For this review, use the dimensioned drawing (mm, ordinates from the lowest corner) and the shaded views. A direction names the side the tool comes from. Give positions to 0.01 mm unless a question says otherwise; leave off trailing zeros. Order: outer loops, then holes, each group sorted by start corner. A loop starts at its lowest first (then second) coordinate and runs counter-clockwise, first axis right, second up. Notation, with made-up numbers: (13, 72) - (30, 72) arc R29 cw to (30, 110) - close; hole circle Ø9 at (12.25, 70). An arc over 180 degrees is marked (long way). One line per item, written item: value.
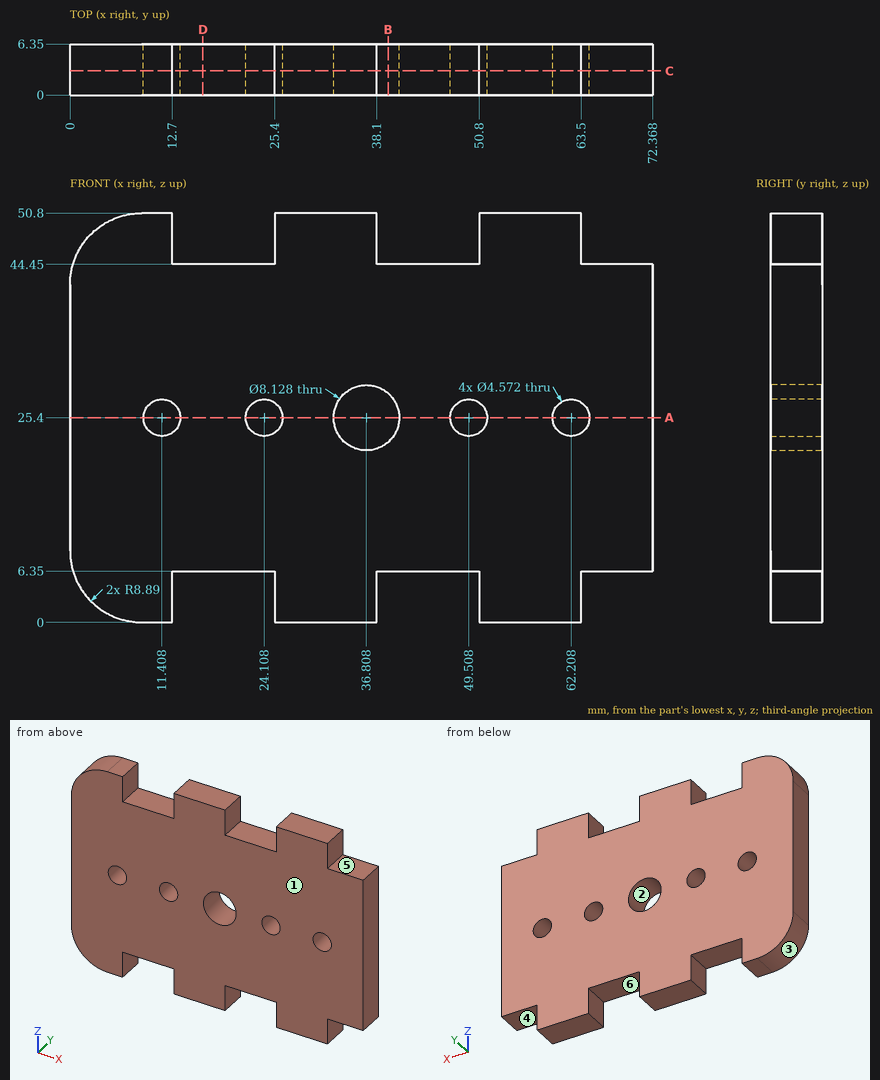
(1) Draft analysis for pull direction X (two halves, no side actions). For the marked faces 1, 2 and 3, state which applies: pulls with the +X half, pulls with the -X half, needs draft (parallel to the pull), parting line crosses it, or undercut.
Answers below:
face 1: needs draft
face 2: undercut
face 3: pulls with the -X half
(2) Take a section at C-C (y = 3). Give the number of separate pieces and of enclosed holes in the cut face, then the cut area to 3 significant figures.
Answers below:
separate pieces: 1
enclosed holes: 5
area: 3,090 mm^2
(3) Take a section at A-A (z = 25.4). Write out the cut boundary in (x, y).
Answers below:
outline: (0, 0) - (9.12, 0) - (9.12, 6.35) - (0, 6.35) - close; (13.69, 0) - (21.82, 0) - (21.82, 6.35) - (13.69, 6.35) - close; (26.39, 0) - (32.74, 0) - (32.74, 6.35) - (26.39, 6.35) - close; (40.87, 0) - (47.22, 0) - (47.22, 6.35) - (40.87, 6.35) - close; (51.79, 0) - (59.92, 0) - (59.92, 6.35) - (51.79, 6.35) - close; (64.49, 0) - (72.37, 0) - (72.37, 6.35) - (64.49, 6.35) - close
(4) Take a section at D-D (x = 16.5). Write out the cut boundary in (y, z), then the cut area to 3 significant figures.
Answers below:
outline: (0, 6.35) - (6.35, 6.35) - (6.35, 44.45) - (0, 44.45) - close
area: 242 mm^2
(5) Wall thickness on line 1 (X direction, y = 2.25, z = 25.4); line 2 (X direction, y = 3, z = 5.5); line 3 (Z direction, x = 68, y = 2): over which ranges is each line inside the solid? List them lowest first. Write a range as from..to.
Answers below:
line 1: x = 0..9.12, 13.69..21.82, 26.39..32.74, 40.87..47.22, 51.79..59.92, 64.49..72.37
line 2: x = 0.67..12.7, 25.4..38.1, 50.8..63.5
line 3: z = 6.35..44.45
(6) Machinability: for the marked faces 4, 5 and 6, which of the approach directions +Z, -Z, +X, -X, +Y, -Y give a long, thin tool a straight path to every point of the face, cutting with its end or side? Answer none if there is none.
Answers below:
face 4: -Z, +X, +Y, -Y
face 5: +Z, +X, +Y, -Y
face 6: -Z, +Y, -Y
(7) For P1, Ø3, axis at y = 4, z = 3.5, coming from the +X side; P2, Ø1.9, axis at x = 43.5, y = 4, coming from the +Z side, all flat-tipped, find the tip position at first contact; note any pin that passes through.
Answers below:
P1: stops at x = 63.5
P2: stops at z = 44.45
(8) Take a section at B-B (x = 39.5). Write out the cut boundary in (y, z).
Answers below:
outline: (0, 6.35) - (6.35, 6.35) - (6.35, 22.36) - (0, 22.36) - close; (0, 28.44) - (6.35, 28.44) - (6.35, 44.45) - (0, 44.45) - close
